from build123d import *

# Parameters (mm, degrees)
F0_W     = 137
F0_H     = 90.5
F0_W_2   = 120.5
F0_H_2   = 77.5
F1_DEPTH = 16
F3_W     = 33
F3_H     = 20.2931881964
F3_H_2   = 28.397909285
F3_W_2   = 75
F3_H_3   = 9.5986060599
F3_H_4   = 10.4013939401
F4_DEPTH = 10
F5_SIZE  = 1.49999


# Not quite as in the source:
# - a fillet or chamfer is up to 0.001 mm smaller than in the source, because OpenCascade refuses the exact size
# - a feature names something its author has since deleted; it is built from what else it names


with BuildPart() as f1:
    # F0 (on Top) → F1 (new body)
    with BuildSketch(Plane.XY):
        with Locations((10.3103105978, 18.8386597227)):
            Rectangle(F0_W, F0_H)
        with Locations((10.5603105978, 18.8386597227)):
            Rectangle(F0_W_2, F0_H_2, mode=Mode.SUBTRACT)
    extrude(amount=F1_DEPTH)

    # F3 (on 3pt) → F4 (cut)
    with BuildSketch(Plane.XY.offset(16)):
        with Locations((10.3103105978, 70.7352538208)):
            Rectangle(F3_W, F3_H)
        with Locations((10.3103105978, 46.3897050802)):
            Rectangle(F3_W, F3_H_2)
        Polygon((-6.1896894022, 32.1907504376), (-6.1896894022, 60.5886597227), (-52.6896894022, 60.5886597227), (-52.6896894022, -18.4113402773), (-47.6896894022, -23.4113402773), (-27.1896894022, -23.4113402773), (-27.1896894022, -13.8127342174), (47.8103105978, -13.8127342174), (47.8103105978, -23.4113402773), (68.8103105978, -23.4113402773), (73.8103105978, -18.4113402773), (73.8103105978, 55.5886597227), (68.8103105978, 60.5886597227), (26.8103105978, 60.5886597227), (26.8103105978, 32.1907504376), align=None)
        with Locations((10.3103105978, -18.6120372474)):
            Rectangle(F3_W_2, F3_H_3)
        with Locations((10.3103105978, -28.6120372474)):
            Rectangle(F3_W_2, F3_H_4)
    extrude(amount=-F4_DEPTH, mode=Mode.SUBTRACT)

    # F5 (size 1.5 in the source; OpenCascade refuses exactly that, so slightly less here)
    f5_edges = [f1.edges().sort_by_distance(p)[0] for p in [
        (-52.689689, 21.08866, 16),
        (-29.439689, 60.58866, 16),
        (78.810311, 18.83866, 16),
        (63.310311, -26.41134, 16),
        (52.810311, 64.08866, 16),
        (-32.189689, 64.08866, 16),
        (-58.189689, 18.83866, 16),
        (-42.689689, -26.41134, 16),
        (71.310311, 58.08866, 16),
        (73.810311, 18.58866, 16),
        (71.310311, -20.91134, 16),
        (-50.189689, -20.91134, 16),
        (58.310311, -23.41134, 16),
        (47.810311, 60.58866, 16),
        (-37.439689, -23.41134, 16),
    ]]
    chamfer(f5_edges, length=F5_SIZE)


solid = f1.part
For this review, take the finished solid that the model builds, in its own axes (mm). A direction names the side the tool comes from. Give positions to 0.01 mm unless a question says otherwise; leave off trailing zeros. Order: outer loops, then holes, each group sorted by start corner. A loop starts at its lowest first (then second) coordinate and runs counter-clockwise, first axis right, second up. Notation, with made-up numbers: (-10.5, 69) - (0.5, 69) arc R9 ccw to (0.5, 83) - close; hole circle Ø8 at (51.25, -12.75). An arc over 180 degrees is marked (long way). Answer as a JSON object with one key per item and string values. Group by question number.
Item 1: Take a section at D-D on z = 1.75. Give the boundary of the cut face in (x, y).
Item 2: Draft analysis for pull direction Y (two halves, no side actions). For faces 1 (the flat face through (10, 59, 0)), 2 (the flat face through (-38, -23.411, 10)), state which applies: pulls with the +Y half, pulls with the -Y half, needs draft (parallel to the pull), parting line crosses it, or undercut.
Item 3: Take a section at A-A on y = -15.5. Give the boundary of the cut face in (x, z).
Item 4: Take a section at B-B on x = -25. Give the boundary of the cut face in (y, z), and give its area (3 significant figures).
Item 5: Take a section at C-C on z = 11.75. Give the boundary of the cut face in (x, y), and give its area (3 significant figures).
Item 6: Wall thickness on line 1 along Y through (x, z) = (24.5, 1.5); line 2 along X through (y, z) = (25, 0.5); line 3 along X through (y, z) = (54.5, 6.25): over which ranges is each line inside the solid? List them lowest first.
Item 7: Machinability: for faces 3 (the flat face through (47.81, -25, 11)), 4 (the flat face through (-58.19, 18, 7)), 5 (the flat face through (-49.69, 18, 3)), 6 (the flat face through (26.81, 62, 11)), 7 (the flat face through (48, 60.589, 10)), which of the approach directions +Z, -Z, +X, -X, +Y, -Y give a long, thin tool a straight path to every point of the face, cutting with its end or side? Answer none if there is none.
Reported:
{
 "1": {"outline": "(-58.19, -26.41) - (78.81, -26.41) - (78.81, 64.09) - (-58.19, 64.09) - close; hole (-49.69, -19.91) - (70.81, -19.91) - (70.81, 57.59) - (-49.69, 57.59) - close"},
 "2": {"face 1": "needs draft", "face 2": "undercut"},
 "3": {"outline": "(-58.19, 0) - (-49.69, 0) - (-49.69, 6) - (-52.69, 6) - (-52.69, 14.5) - (-54.19, 16) - (-56.69, 16) - (-58.19, 14.5) - close; (70.81, 0) - (78.81, 0) - (78.81, 14.5) - (77.31, 16) - (75.31, 16) - (73.81, 14.5) - (73.81, 6) - (70.81, 6) - close"},
 "4": {"outline": "(-26.41, 0) - (-19.91, 0) - (-19.91, 6) - (-26.41, 6) - close; (57.59, 0) - (64.09, 0) - (64.09, 14.5) - (62.59, 16) - (62.09, 16) - (60.59, 14.5) - (60.59, 6) - (57.59, 6) - close", "area": "111 mm^2"},
 "5": {"outline": "(-58.19, -26.41) - (-27.19, -26.41) - (-27.19, -23.41) - (-47.69, -23.41) - (-52.69, -18.41) - (-52.69, 60.59) - (-6.19, 60.59) - (-6.19, 64.09) - (-58.19, 64.09) - close; (26.81, 60.59) - (68.81, 60.59) - (73.81, 55.59) - (73.81, -18.41) - (68.81, -23.41) - (47.81, -23.41) - (47.81, -26.41) - (78.81, -26.41) - (78.81, 64.09) - (26.81, 64.09) - close", "area": "1,470 mm^2"},
 "6": {"line 1": "-26.41 to -19.91, 57.59 to 64.09", "line 2": "-58.19 to -49.69, 70.81 to 78.81", "line 3": "-58.19 to -52.69, 73.81 to 78.81"},
 "7": {"face 3": "+Z, -Y", "face 4": "+Z, -Z, -X, +Y, -Y", "face 5": "+Z, -Z", "face 6": "+Z, +Y, -Y", "face 7": "+Z"}
}
